Source: CAD feature listing. Evaluate the final solid. Frame: model axes, mm. Coordinates: 2 decimals unless noted, no trailing zeros. Loops run counter-clockwise (first coordinate to the right, second up) from the corner with the lowest first, then second, coordinate; pieces in that order, holes last.
Item 1: Section query C-C, the plane z = 17.5. Return the cut outline in (x, y).
Item 2: Pin query (flat end, axial travel): pin 1 Ø1 at (y, z) = (-41, 9.5) entering from +X; pin 2 Ø2 at (x, y) = (104, -9) entering from -Z; pin 3 Ø10 at (y, z) = (-9.5, 7.5) entering from -X. Return the tip coordinate at first contact, or that it passes through.
Item 3: Section query A-A, the plane y = -34.5. Return the cut outline in (x, z).
Item 4: Section query B-B, the plane x = 46.5. Return the cut outline in (y, z).
Item 5: Line query: probe 1 along Z at (x, y) = (89.5, -29.5); probe 2 along Z at (x, y) = (4.5, -9); probe 3 along X at (y, z) = (-8.5, 11). Output: solid intervals per line, ascending.
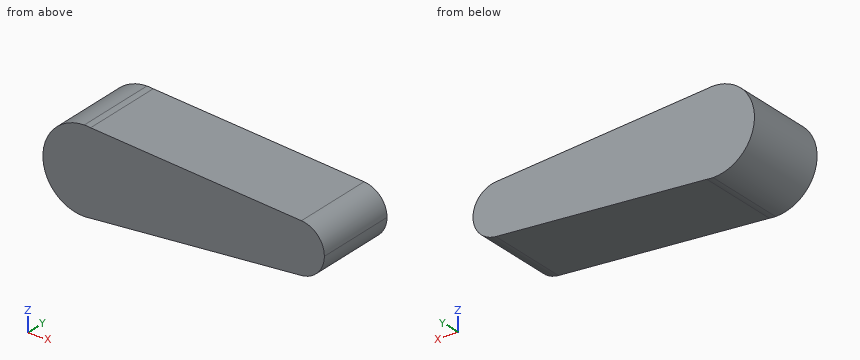
```python
from build123d import *

# Parameters (mm, degrees)
F1_DEPTH = 50


with BuildPart() as f1:
    # F0 (on Front) → F1 (new body)
    with BuildSketch(Plane.XZ):
        with BuildLine():
            Line((3.806931, 24.708445), (0, 25))
            ThreePointArc((0, 25), (-25, 0), (0, -25))
            Line((0, -25), (3.806931, -24.708445))
            ThreePointArc((3.806931, -24.708445), (18.975949, -16.276159), (25, 0))
            ThreePointArc((25, 0), (18.975949, 16.276159), (3.806931, 24.708445))
        make_face()
        with BuildLine():
            ThreePointArc((3.806931, 24.708445), (1.909039, 24.927005), (0, 25))
            Line((0, 25), (3.806931, 24.708445))
        make_face()
        with BuildLine():
            Line((3.806931, -24.708445), (0, -25))
            ThreePointArc((0, -25), (1.909039, -24.927005), (3.806931, -24.708445))
        make_face()
        with BuildLine():
            Line((131.145424, 14.956203), (3.806931, 24.708445))
            ThreePointArc((3.806931, 24.708445), (18.975949, 16.276159), (25, 0))
            ThreePointArc((25, 0), (18.975949, -16.276159), (3.806931, -24.708445))
            Line((3.806931, -24.708445), (131.145424, -14.956203))
            ThreePointArc((131.145424, -14.956203), (115, 0), (131.145424, 14.956203))
        make_face()
        with BuildLine():
            ThreePointArc((145, 0), (141.004121, 10.193592), (131.145424, 14.956203))
            ThreePointArc((131.145424, 14.956203), (115, 0), (131.145424, -14.956203))
            ThreePointArc((131.145424, -14.956203), (141.004121, -10.193592), (145, 0))
        make_face()
    extrude(amount=F1_DEPTH)


solid = f1.part
```
Verdict:
1. outline: (-17.85, -50) - (97.93, -50) - (97.93, 0) - (-17.85, 0) - close
2. pin 1: stops at x = 142
2. pin 2: stops at z = -17.11
2. pin 3: stops at x = -24.87
3. outline: (0, -25) arc R25 ccw to (3.81, -24.71) - (131.15, -14.96) arc R15 ccw to (131.15, 14.96) - (3.81, 24.71) arc R25 ccw to (0, 25) arc R25 ccw to start
4. outline: (-50, -21.44) - (0, -21.44) - (0, 21.44) - (-50, 21.44) - close
5. probe 1: z = -18.15 to 18.15
5. probe 2: z = -24.66 to 24.66
5. probe 3: x = -22.45 to 140.2
